Check sheet for the modelled part. Datum: model origin and axes. Units: mm. A direction names the side the tool comes from. Give positions to 0.01 mm unless a question says otherwise; leave off trailing zeros. Order: outer loops, then holes, each group sorted by start corner. A loop starts at its lowest first (then second) coordinate and runs counter-clockwise, first axis right, second up. Notation, with made-up numbers: (-18.5, 46.5) -> (21.5, 46.5) arc R19 cw to (21.5, 68.5) -> close; hole circle Ø10 at (42.5, 32.5). An arc over 180 degrees is marked (long way). Write each question's results on one line, items separated by ' | '.
from build123d import *

# Parameters (mm, degrees)
F0_W     = 6.35
F0_H     = 7.62
F1_DEPTH = 12.7
F3_DEPTH = 2.54
F5_DEPTH = 2.54


with BuildPart() as f1:
    # F0 (on Top) → F1 (new body)
    with BuildSketch(Plane.XY):
        with Locations((3.175, -3.81)):
            Rectangle(F0_W, F0_H)
    extrude(amount=F1_DEPTH)

    # F2 (on face) → F3 (join)
    with BuildSketch(Plane.YZ.offset(6.35)):
        with BuildLine():
            Line((-5.715, 6.35), (-3.81, 6.35))
            Line((-3.81, 6.35), (-1.905, 6.35))
            ThreePointArc((-1.905, 6.35), (-3.81, 8.255), (-5.715, 6.35))
        make_face()
        with BuildLine():
            Line((-1.905, 6.35), (-3.81, 6.35))
            Line((-3.81, 6.35), (-5.715, 6.35))
            ThreePointArc((-5.715, 6.35), (-3.81, 4.445), (-1.905, 6.35))
        make_face()
    extrude(amount=F3_DEPTH)

    # F4 (on face) → F5 (join)
    with BuildSketch(Plane(origin=(0, 0, 0), x_dir=(0, -1, 0), z_dir=(-1, 0, 0))):
        with BuildLine():
            Line((1.905, 6.35), (3.81, 6.35))
            Line((3.81, 6.35), (5.715, 6.35))
            ThreePointArc((5.715, 6.35), (3.81, 8.255), (1.905, 6.35))
        make_face()
        with BuildLine():
            Line((5.715, 6.35), (3.81, 6.35))
            Line((3.81, 6.35), (1.905, 6.35))
            ThreePointArc((1.905, 6.35), (3.81, 4.445), (5.715, 6.35))
        make_face()
    extrude(amount=F5_DEPTH)


solid = f1.part
1. Gauge pin test, flat ends, axial feed: pin 1 Ø4 at (x, y) = (-1, -4.5) entering from -Z; pin 2 Ø1.5 at (y, z) = (-6, 1.5) entering from +X; pin 3 Ø2.5 at (y, z) = (-4.5, 9.5) entering from -X. Record the tip position at first contact, or that the pin passes through.
Verdict:
pin 1: stops at z = 0 | pin 2: stops at x = 6.35 | pin 3: stops at x = 0
2. Section check C-C on z = 1. Record the cut outline in (x, y), then the cut area to 3 significant figures.
Verdict:
outline: (0, -7.62) -> (6.35, -7.62) -> (6.35, 0) -> (0, 0) -> close | area: 48.4 mm^2
3. Section check A-A on z = 6.35. Record the cut outline in (x, y) (3 decimals).
Verdict:
outline: (-2.54, -5.715) -> (0, -5.715) -> (0, -7.62) -> (6.35, -7.62) -> (6.35, -5.715) -> (8.89, -5.715) -> (8.89, -1.905) -> (6.35, -1.905) -> (6.35, 0) -> (0, 0) -> (0, -1.905) -> (-2.54, -1.905) -> close
4. Material ranges on probe 1 along X at (y, z) = (-4, 10); probe 2 along Z at (x, y) = (7.5, -3.75); probe 3 along Z at (x, y) = (-1.5, -3.25), recorded low to high. Write a range as from..to.
Verdict:
probe 1: x = 0..6.35 | probe 2: z = 4.45..8.25 | probe 3: z = 4.53..8.17
5. Section check D-D on y = -6. Record the cut outline in (x, z), then the cut area to 3 significant figures.
Verdict:
outline: (0, 0) -> (6.35, 0) -> (6.35, 12.7) -> (0, 12.7) -> close | area: 80.6 mm^2
6. Section check B-B on y = -3.81. Record the cut outline in (x, z) (3 decimals).
Verdict:
outline: (-2.54, 4.445) -> (0, 4.445) -> (0, 0) -> (6.35, 0) -> (6.35, 4.445) -> (8.89, 4.445) -> (8.89, 8.255) -> (6.35, 8.255) -> (6.35, 12.7) -> (0, 12.7) -> (0, 8.255) -> (-2.54, 8.255) -> close
7. Access from +Z, -Z, +X, -X, +Y, -Y to the whole of each face (thin tool, end or side, straight path). Record for faces 1 (the cylindrical face through (-1.25, -2.93, 8.04)), 2 (the cylindrical face through (7.6, -4.69, 8.04)), 3 (the flat face through (8.89, -4, 6)).
Verdict:
face 1: -X | face 2: +X | face 3: +Z, -Z, +X, +Y, -Y
